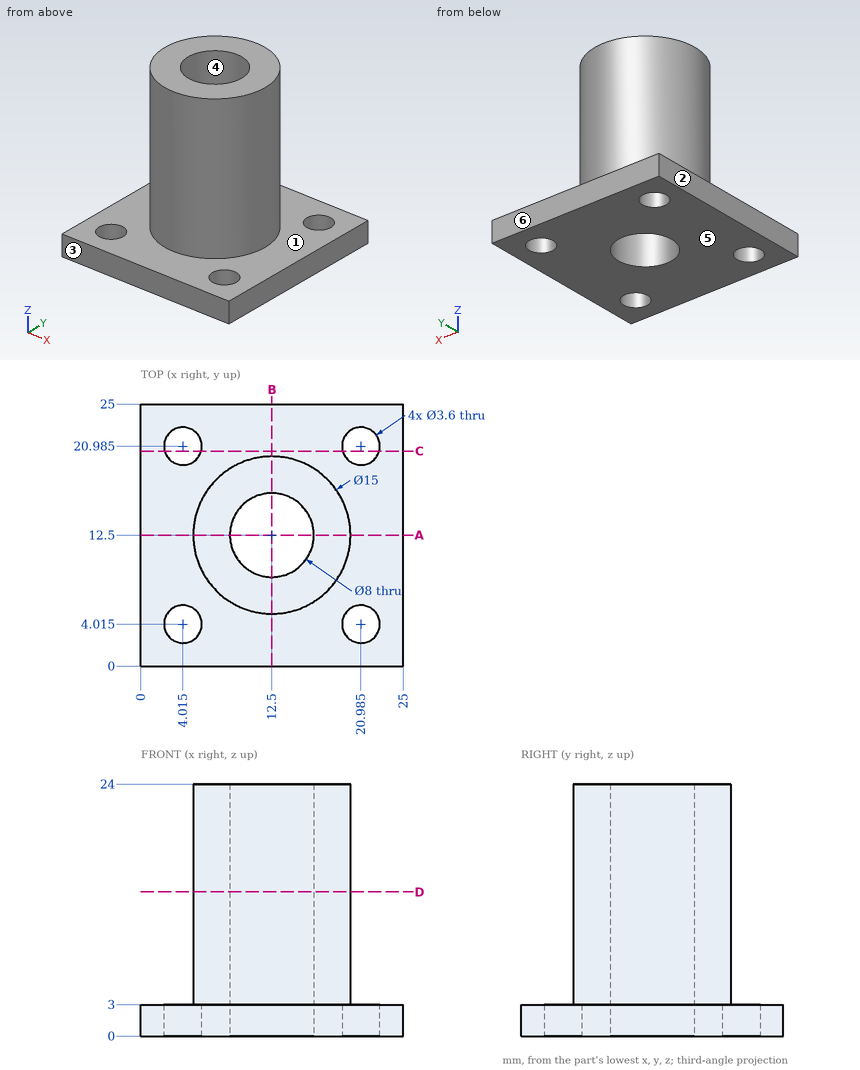
Job drawing, mm, ordinate dimensions from the low corner. One solid piece. A direction names the side the tool comes from. Coordinates: 2 decimals unless noted, no trailing zeros. Order: outer loops, then holes, each group sorted by start corner. A loop starts at its lowest first (then second) coordinate and runs counter-clockwise, first axis right, second up. Notation, with made-up numbers: M -15,29.25 L 21,29.25 A4 cw 21,35.25 Z; hole C 33,12.5 d5. An arc over 180 degrees is marked long. Return JSON: item names as keys, results as strings.
1. Saw through at D-D (z = 13.75). Give the cut face in (x, y), and give its area (3 significant figures).
Ans:
{"outline": "C 12.5,12.5 d15; hole C 12.5,12.5 d8", "area": "126 mm^2"}
2. Drill centre lines: probe 1 along X at (y, z) = (19.5, 2.5); probe 2 along Y at (x, z) = (10.5, 11.75) (1 decimal). Where is each one in solid material? Low to high.
Ans:
{"probe 1": "0 to 3, 5.03 to 19.97, 22 to 25", "probe 2": "5.3 to 9, 16 to 19.7"}
3. Flat gauge pins, fed straight in: pin 1 (2 mm diameter, centred on x = 6, z = 11, fed in from +Y); pin 2 (8 mm diameter, centred on x = 4.5, z = 19.5, fed in from +Y) (1 decimal); pin 3 (5 mm diameter, centred on x = 10.5, z = 21, fed in from +Y); pin 4 (3 mm diameter, centred on x = 4.01, y = 20.99, fed in from -Z). Where does each tip first touch, or does it go through?
Ans:
{"pin 1": "y = 17.6", "pin 2": "y = 18.8", "pin 3": "y = 20", "pin 4": "through"}
4. Pull direction Y, two halves, no side cores. Call the marked faces 3, 4, 5 and 6: +Y half, -Y half, draft (parallel to the pull), parting line (faces both ways), or undercut.
Ans:
{"face 3": "-Y half", "face 4": "undercut", "face 5": "draft", "face 6": "+Y half"}
5. Saw through at C-C (y = 20.5). Give the cut face in (x, z).
Ans:
{"outline": "M 0,0 L 2.28,0 L 2.28,3 L 0,3 Z; M 5.75,0 L 19.25,0 L 19.25,3 L 5.75,3 Z; M 22.72,0 L 25,0 L 25,3 L 22.72,3 Z"}
6. Tool access for the marked faces 1 and 2: list every direction of +Z, -Z, +X, -X, +Y, -Y with a clear straight run to the whole face (end or side of a thin tool).
Ans:
{"face 1": "+Z", "face 2": "+Z, -Z, -X, +Y, -Y"}
7. Saw through at A-A (y = 12.5). Give the cut face in (x, z).
Ans:
{"outline": "M 0,0 L 8.5,0 L 8.5,24 L 5,24 L 5,3 L 0,3 Z; M 16.5,0 L 25,0 L 25,3 L 20,3 L 20,24 L 16.5,24 Z"}
